Geometry: final body of the model. Coordinates: model frame, mm. Round coordinates to 2 decimals unless told otherwise and drop trailing zeros. Loops run counter-clockwise (first coordinate to the right, second up) from the corner with the lowest first, then second, coordinate; pieces in that order, holes last. Notation, with made-up numbers: (-26, 8.25) -> (24, 8.25) arc R17 ccw to (24, 19.25) -> close; hole circle Ø9 at (36.5, -14). An arc over 180 degrees is marked (long way). Answer in a Markdown table with one row per item.
```python
from build123d import *

# Parameters (mm, degrees)
SCHIZZO1_W                   = 140
SCHIZZO1_H                   = 80
SCHIZZO1_R                   = 3.5
SCHIZZO1_W_2                 = 95
SCHIZZO1_H_2                 = 61
ESTRUSIONE_ESTRUSIONE1_DEPTH = 3
SCHIZZO2_W                   = 7
SCHIZZO2_H                   = 4
ESTRUSIONE_ESTRUSIONE2_DEPTH = 3
RIPETIZIONE_A_L1_COUNT       = 10
RIPETIZIONE_A_L1_PITCH       = 14
SCHIZZO3_W                   = 4
SCHIZZO3_H                   = 5.714285714
ESTRUSIONE_ESTRUSIONE3_DEPTH = 3
RIPETIZIONE_A_L2_COUNT       = 7
RIPETIZIONE_A_L2_PITCH       = 11.428571429
SCHIZZO4_W                   = 95
SCHIZZO4_H                   = 61
SCHIZZO4_W_2                 = 84.5
SCHIZZO4_H_2                 = 57
ESTRUSIONE_ESTRUSIONE4_DEPTH = 3


with BuildPart() as part:
    # Schizzo1 → Estrusione-Estrusione1 (new body)
    with BuildSketch(Plane.XY):
        with Locations((70, 40)):
            Rectangle(SCHIZZO1_W, SCHIZZO1_H)
        with Locations((123, 42.5)):
            Circle(SCHIZZO1_R, mode=Mode.SUBTRACT)
        with Locations((59.5, 39.5)):
            Rectangle(SCHIZZO1_W_2, SCHIZZO1_H_2, mode=Mode.SUBTRACT)
    extrude(amount=ESTRUSIONE_ESTRUSIONE1_DEPTH)

    # Schizzo2 → Estrusione-Estrusione2 (add)
    with BuildSketch(Plane.XY.offset(3)):
        with Locations((7, 82)):
            Rectangle(SCHIZZO2_W, SCHIZZO2_H)
        with Locations((7, -2)):
            Rectangle(SCHIZZO2_W, SCHIZZO2_H)
    estrusione_estrusione2 = extrude(amount=-ESTRUSIONE_ESTRUSIONE2_DEPTH)

    # Ripetizione a L1: Estrusione-Estrusione2 ×10
    with Locations(*[(i * RIPETIZIONE_A_L1_PITCH, 0, 0) for i in range(1, RIPETIZIONE_A_L1_COUNT)]):
        add(estrusione_estrusione2)

    # Schizzo3 → Estrusione-Estrusione3 (add)
    with BuildSketch(Plane.XY.offset(3)):
        with Locations((-2, 74.285714286)):
            Rectangle(SCHIZZO3_W, SCHIZZO3_H)
        with Locations((142, 74.285714286)):
            Rectangle(SCHIZZO3_W, SCHIZZO3_H)
    estrusione_estrusione3 = extrude(amount=-ESTRUSIONE_ESTRUSIONE3_DEPTH)

    # Ripetizione a L2: Estrusione-Estrusione3 ×7
    with Locations(*[(0, -i * RIPETIZIONE_A_L2_PITCH, 0) for i in range(1, RIPETIZIONE_A_L2_COUNT)]):
        add(estrusione_estrusione3)

    # Schizzo4 → Estrusione-Estrusione4 (add)
    with BuildSketch(Plane.XY.offset(3)):
        with Locations((59.5, 39.5)):
            Rectangle(SCHIZZO4_W, SCHIZZO4_H)
        with Locations((57.25, 39.5)):
            Rectangle(SCHIZZO4_W_2, SCHIZZO4_H_2, mode=Mode.SUBTRACT)
    extrude(amount=-ESTRUSIONE_ESTRUSIONE4_DEPTH)


solid = part.part
```
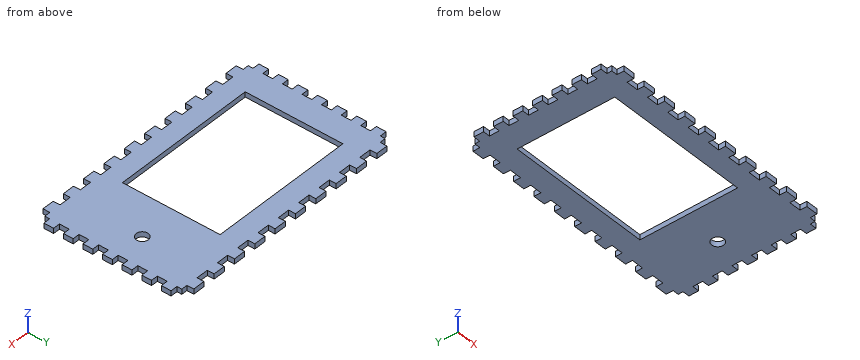
Item 1: Section query A-A, the plane y = 34. Output: boundary loops of the cut face in (x, z).
Ans:
| item | result |
|---|---|
| outline | (0, 0) -> (15, 0) -> (15, 3) -> (0, 3) -> close; (99.5, 0) -> (140, 0) -> (140, 3) -> (99.5, 3) -> close |
Item 2: Section query B-B, the plane x = 93. Output: boundary loops of the cut face in (y, z).
Ans:
| item | result |
|---|---|
| outline | (-4, 0) -> (11, 0) -> (11, 3) -> (-4, 3) -> close; (68, 0) -> (84, 0) -> (84, 3) -> (68, 3) -> close |
Item 3: Ray query, L1, parallel to X at y = 56, z = 0.2; L2, parallel to Y at x = 123, z = 1.5; L3, parallel to X at y = 49, z = 0.2. Return the intervals inside material, ascending.
Ans:
| item | result |
|---|---|
| L1 | 0 to 15, 99.5 to 140 |
| L2 | 0 to 39, 46 to 80 |
| L3 | -4 to 15, 99.5 to 144 |
Item 4: First-contact query: P1, Ø1.5, axis at x = 84.5, z = 1.5, coming from the -Y side; P2, Ø0.9, axis at x = -2.5, z = 1, coming from the -Y side; P3, Ø0.9, axis at y = 82.5, z = 1, coming from the -X side. Flat tips, straight axial feed; report the tip coordinate or a pass-through.
Ans:
| item | result |
|---|---|
| P1 | y = 0 |
| P2 | y = 2.86 |
| P3 | x = 3.5 |
Item 5: Section query C-C, the plane z = 1.85. State how many separate pieces and enclosed holes the cut face has, and give its area (4 significant figures).
Ans:
| item | result |
|---|---|
| separate pieces | 1 |
| enclosed holes | 2 |
| area | 7,225 mm2 |
